The listing builds one solid part. Answer for the finished solid, in the listing's coordinates (mm). Face numbers are marked on the shaded views. Give positions to 0.01 mm unless a question says otherwise; leave off trailing zeros. Loops run counter-clockwise (first coordinate to the right, second up) from the corner with the lowest first, then second, coordinate; pieces in that order, holes last. Notation, with made-up numbers: M -14.5,8.25 L 36.5,8.25 A21 cw 36.5,37.25 Z; hole C -11,-11 d11. An arc over 180 degrees is marked long. Return JSON: item names as keys, results as strings.
from build123d import *

# Parameters (mm, degrees)
SKETCH_1_R          = 12
EXTRUDE_1_DEPTH     = 5
SKETCH_2_R          = 7.5
CUT_EXTRUDE_1_DEPTH = 6
SKETCH_3_R          = 11.075
SKETCH_3_R_2        = 8.4
CUT_EXTRUDE_2_DEPTH = 0.5
SKETCH_4_R          = 11.075
SKETCH_4_R_2        = 8.4
CUT_EXTRUDE_3_DEPTH = 0.5


with BuildPart() as part:
    # 草圖1 → 填料-伸長1 (new body)
    with BuildSketch(Plane.XY):
        Circle(SKETCH_1_R)
    extrude(amount=EXTRUDE_1_DEPTH)

    # 草圖2 → 除料-伸長1 (cut, through all)
    with BuildSketch(Plane.XY.offset(5)):
        Circle(SKETCH_2_R)
    extrude(amount=-CUT_EXTRUDE_1_DEPTH, mode=Mode.SUBTRACT)

    # 草圖3 → 除料-伸長2 (cut)
    with BuildSketch(Plane.XY.offset(5)):
        Circle(SKETCH_3_R)
        Circle(SKETCH_3_R_2, mode=Mode.SUBTRACT)
    extrude(amount=-CUT_EXTRUDE_2_DEPTH, mode=Mode.SUBTRACT)

    # 草圖4 → 除料-伸長3 (cut)
    with BuildSketch(Plane(origin=(0, 0, 0), x_dir=(-1, 0, 0), z_dir=(0, 0, -1))):
        Circle(SKETCH_4_R)
        Circle(SKETCH_4_R_2, mode=Mode.SUBTRACT)
    extrude(amount=-CUT_EXTRUDE_3_DEPTH, mode=Mode.SUBTRACT)


solid = part.part
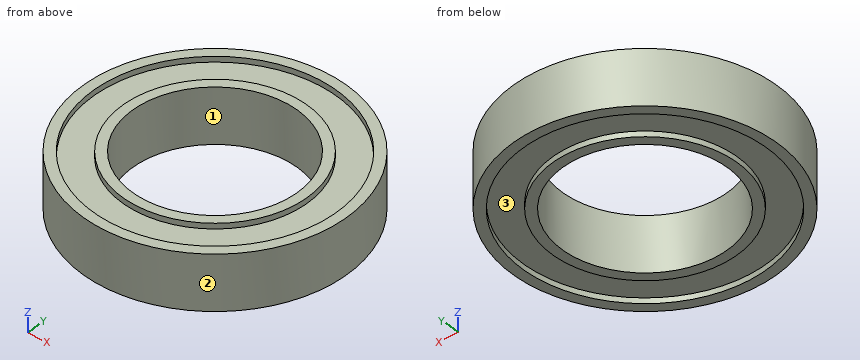
(1) Given pin 1 (2 mm diameter, centred on x = -1.5, z = 2, fed in from -Y); pin 2 (2 mm diameter, centred on x = -2, z = 3, fed in from +Y), each flat-ended and moving along its own axis, determine where each tip first touches the part or whether it passes through.
Values follow:
{"pin 1": "y = -11.99", "pin 2": "y = 11.96"}
(2) Determine the mould class of the marked faces 1, 2 and 3 for opening direction Y: released by +Y, released by -Y, zero draft, split by the parting line, or undercut.
Values follow:
{"face 1": "undercut", "face 2": "split by the parting line", "face 3": "undercut"}
(3) The part is cut by section A-A (y = 0). Determine the outline of the cut face in (x, z) (3 decimals), and give its area (4 significant figures).
Values follow:
{"outline": "M -12,0 L -11.075,0 L -11.075,0.5 L -8.4,0.5 L -8.4,0 L -7.5,0 L -7.5,5 L -8.4,5 L -8.4,4.5 L -11.075,4.5 L -11.075,5 L -12,5 Z; M 7.5,0 L 8.4,0 L 8.4,0.5 L 11.075,0.5 L 11.075,0 L 12,0 L 12,5 L 11.075,5 L 11.075,4.5 L 8.4,4.5 L 8.4,5 L 7.5,5 Z", "area": "39.65 mm²"}
(4) Straight lines are drawn through the part: line 1 along Y through (x, z) = (0, 0.1) (3 decimals); line 2 along Y through (x, z) = (0, 2.8); line 3 along X through (y, z) = (-5.5, 4.65). For each, find the intervals that lie inside material, in ascending order.
Values follow:
{"line 1": "-12 to -11.075, -8.4 to -7.5, 7.5 to 8.4, 11.075 to 12", "line 2": "-12 to -7.5, 7.5 to 12", "line 3": "-10.67 to -9.61, -6.35 to -5.1, 5.1 to 6.35, 9.61 to 10.67"}
(5) The part is cut by section C-C (z = 1.55). Determine the outline of the cut face in (x, y), and give its area (3 significant figures).
Values follow:
{"outline": "C 0,0 d24; hole C 0,0 d15", "area": "276 mm²"}
(6) The part is cut by section D-D (y = -8). Determine the outline of the cut face in (x, z).
Values follow:
{"outline": "M -8.94,0 L -7.66,0 L -7.66,0.5 L -2.56,0.5 L -2.56,0 L 2.56,0 L 2.56,0.5 L 7.66,0.5 L 7.66,0 L 8.94,0 L 8.94,5 L 7.66,5 L 7.66,4.5 L 2.56,4.5 L 2.56,5 L -2.56,5 L -2.56,4.5 L -7.66,4.5 L -7.66,5 L -8.94,5 Z"}
